Verification items for the finished model (mm, model axes). A direction names the side the tool comes from. Round coordinates to 2 decimals unless told otherwise and drop trailing zeros. Order: outer loops, then holes, each group sorted by start corner. A loop starts at its lowest first (then second) coordinate and runs counter-clockwise, first axis right, second up. Notation, with made-up numbers: M -7,-26.5 L 21,-26.5 A29 cw 21,4.5 Z; hole C -35,12.5 d3. An arc over 180 degrees is marked long. Use CSV: the item, a comma, the result in double quotes. Start each with the question number.
Q1. Sectioned sample at A-A (x = -865). Enter the section's corners in (y, z).
Q2. Sectioned sample at C-C (z = -13.5). Enter the section's corners in (x, y).
Q3. Set-up check for faces 4 (the face through (-990.6, 5, -2)), 5 (the face through (-488, 2.54, -11)): record each of +Z, -Z, +X, -X, +Y, -Y from which the full face is reachable in a straight line by a thin tool's end or side.
Q4. Sectioned sample at B-B (y = 13.5). Enter the section's corners in (x, z), and give its area (3 significant figures).
Q5. Gauge pin test, flat ends, axial feed: pin 1 Ø2 at (x, y) = (-471.5, 10) entering from -Z; pin 2 Ø5 at (x, z) = (-443.5, -12.5) entering from +Y. Record the tip position at first contact, or that the pin passes through.
Q6. Mould release check, pull along Z, two halves, no side actions. Record for faces 1 (the face through (-488, 11, -2.54)), 2 (the face through (-488, 9, 0)), 3 (the face through (0, 5, -2)): +Z half, -Z half, draft (parallel to the pull), parting line (faces both ways), or undercut.
Q7. Scan lines: line 1 (Y direction, x = -739.5, z = -13.75); line 2 (Z direction, x = -913, y = 16.5). Record each from-to range of solid material in increasing order.
Autodesk Inventor part; units mm, degrees
ref_plane "YZ Plane" through (0, 0, 0) normal (1, 0, 0) x (0, 1, 0)
ref_plane "XZ Plane" through (0, 0, 0) normal (0, 1, 0) x (-1, 0, 0)
ref_plane "XY Plane" through (0, 0, 0) normal (0, 0, 1) x (1, 0, 0)
sketch "Sketch1" plane through (0, 0, 0) normal (1, 0, 0) x (0, 1, 0)
  line L0 (0, 0) -> (0, -19.05)
  line L1 (0, 0) -> (19.05, 0)
  line L2 (19.05, -2.54) -> (2.54, -2.54)
  line L3 (2.54, -2.54) -> (2.54, -19.05)
  line L4 (2.54, -19.05) -> (0, -19.05)
  line L5 (19.05, 0) -> (19.05, -2.54)
  dimension "d0" = 19.05
  dimension "d2" = 19.05
  dimension "d3" = 2.54
extrude "Extrusion1" add sketch "Sketch1" against normal blind 990.6
properties part number "AluminumLchannel"
Verdict:
1,outline,"M 0,-19.05 L 2.54,-19.05 L 2.54,-2.54 L 19.05,-2.54 L 19.05,0 L 0,0 Z"
2,outline,"M -990.6,0 L 0,0 L 0,2.54 L -990.6,2.54 Z"
3,face 4,"+Z, -Z, -X, +Y, -Y"
3,face 5,"-Z, +X, -X, +Y"
4,outline,"M -990.6,-2.54 L 0,-2.54 L 0,0 L -990.6,0 Z"
4,area,"2,520 mm²"
5,pin 1,"stops at z = -2.54"
5,pin 2,"stops at y = 2.54"
6,face 1,"-Z half"
6,face 2,"+Z half"
6,face 3,"draft"
7,line 1,"y = 0 to 2.54"
7,line 2,"z = -2.54 to 0"
